Check sheet for the modelled part. Datum: model origin and axes. Units: mm. Face numbers are marked on the shaded views. Give positions to 0.01 mm unless a question says otherwise; leave off trailing zeros. Order: outer loops, then holes, each group sorted by start corner. A loop starts at its lowest first (then second) coordinate and runs counter-clockwise, first axis right, second up.
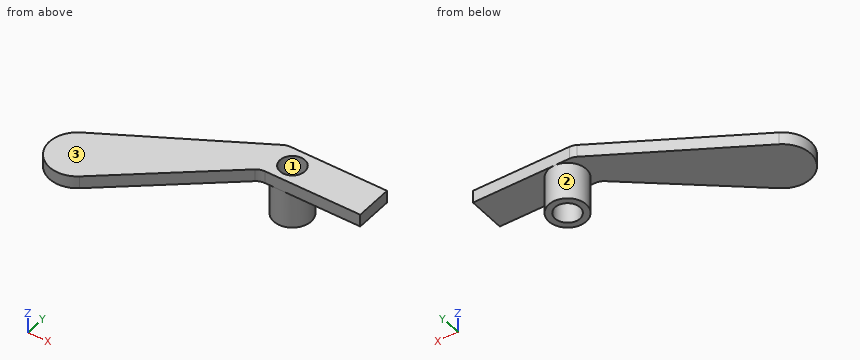
Autodesk Inventor part; units mm, degrees
ref_plane "YZ Plane" through (0, 0, 0) normal (1, 0, 0) x (0, 1, 0)
ref_plane "XZ Plane" through (0, 0, 0) normal (0, 1, 0) x (-1, 0, 0)
ref_plane "XY Plane" through (0, 0, 0) normal (0, 0, 1) x (1, 0, 0)
sketch "Skizze1" plane through (0, 0, 0) normal (0, 0, 1) x (1, 0, 0)
  line L0 (0, 0) -> (0, 6)
  line L1 (0, 6) -> (-23.3827, -7.5)
  arc A0 (-23.3827, -7.5) -> (-18.3295, -14.9173) centre (-21.1327, -11.3971) ccw
  line L2 (-18.3295, -14.9173) -> (0, 0)
  line L3 (0, 6) -> (16, 6)
  line L4 (16, 6) -> (16, 0)
  line L5 (16, 0) -> (0, 0)
  line L6 (-21.1327, -11.3971) -> (0, 3) construction
  dimension "d1" = 6
  dimension "d3" = 30
  dimension "d4" = 4.5
  dimension "d5" = 16
  dimension "d6" = 27
extrude "Extrusion1" add sketch "Skizze1" along normal mid plane 2
sketch "Skizze2" plane through (0, 0, -1) normal (0, 0, -1) x (-1, 0, 0)
  circle A0 centre (-3, 3) radius 3
  line L0 (-16, 6) -> (-16, 0)
  point P0 (0, 0)
  point P1 (-16, 3)
  dimension "d9" = 6
  dimension "d10" = 13
extrude "Extrusion2" add sketch "Skizze2" along normal blind 6
sketch "Skizze3" plane through (3, 3, -7) normal (0, 0, -1) x (-1, 0, 0)
  circle A0 centre (0, 0) radius 3
  point P0 (3, -3)
hole "Bohrung1" at (3, 3, -7) direction (0, 0, 1) diameter 4 depth 8
fillet "Rundung1" radius 2 2 edges at (0, 6, 0) (0, 0, 0)
properties part number "1 part 12"
Q1. Sectioned sample at B-B, the plane y = 3.75. Record the cut outline in (x, z), plus the area to 3 significant figures.
Q2. Material ranges on line 1 (Y direction, x = 3, z = -3.75); line 2 (Z direction, x = -7, y = -1), recorded low to high.
Q3. Sectioned sample at C-C, the plane x = 7.5. Record the cut outline in (y, z).
Q4. Draft check along X on the marked faces 1, 2 and 3. Enter one of: pulls with the +X half, pulls with the -X half, needs draft (parallel to the pull), parting line crosses it, or undercut.
Q5. Go/stop test with flat-tipped pins: P1, Ø1.5, axis at x = -18.5, z = -1.5, coming from the -Y side; P2, Ø2, axis at x = -15.5, y = -1.5, coming from the +Z side; P3, Ø1.6, axis at x = 11.5, z = -0.5, coming from the -Y side; P4, Ø6.5, axis at x = -17.5, y = -6.5, coming from the -Z side. Record where each tip stops, or that it passes through.
Q6. Sectioned sample at A-A, the plane z = 0. Record the cut outline in (x, y).
Q7. Sectioned sample at D-D, the plane y = -4.75. Record the cut outline in (x, z).
Filled in:
1. outline: (-3.9, -1) - (0.1, -1) - (0.1, -7) - (1.15, -7) - (1.15, 1) - (-3.9, 1) - close; (4.85, -7) - (5.9, -7) - (5.9, -1) - (16, -1) - (16, 1) - (4.85, 1) - close
1. area: 45.0 mm2
2. line 1: y = 0 to 1, 5 to 6
2. line 2: z = -1 to 1
3. outline: (0, -1) - (6, -1) - (6, 1) - (0, 1) - close
4. face 1: undercut
4. face 2: parting line crosses it
4. face 3: needs draft
5. P1: stops at y = -15.39
5. P2: passes through
5. P3: stops at y = 0
5. P4: stops at z = -1
6. outline: (-23.38, -7.5) arc R4.5 ccw (long way) to (-18.33, -14.92) - (-0.55, -0.45) arc R2 cw to (0.71, 0) - (16, 0) - (16, 6) - (0.54, 6) arc R2 ccw to (-0.46, 5.73) - close; hole circle Ø4 at (3, 3)
7. outline: (-18.62, -1) - (-5.84, -1) - (-5.84, 1) - (-18.62, 1) - close
